Work out the finished part from the listing and answer in its coordinate system (mm). Round coordinates to 2 decimals unless told otherwise and drop trailing zeros. Order: outer loops, then holes, each group sorted by start corner. A loop starts at its lowest first (then second) coordinate and runs counter-clockwise, first axis right, second up. Notation, with made-up numbers: (14.25, 0.5) - (19.25, 0.5) arc R28 cw to (19.25, 20.5) - close; hole circle Ø10 at (50, 46.25). An arc over 180 degrees is marked (long way). Use CSV: the item, a comma, the result in double quotes.
from build123d import *

# Parameters (mm, degrees)
SKETCH1_R             = 20
SKETCH1_R_2           = 1
SKETCH1_R_3           = 5
BOSS_EXTRUDE1_DEPTH   = 9.35
M4X0_7_TAPPED_HOLE1_D = 3.3


with BuildPart() as part:
    # Sketch1 → Boss-Extrude1 (new body)
    with BuildSketch(Plane(origin=(0, 0, 0), x_dir=(1, 0, 0), z_dir=(0, 1, 0))):
        with Locations(Location((0, 0, 0), (0, 0, 270))):
            Circle(SKETCH1_R)
        with Locations(Location((0, 10, 0), (0, 0, 270))):
            Circle(SKETCH1_R_2, mode=Mode.SUBTRACT)
        with Locations(Location((8.660254038, 5, 0), (0, 0, 270))):
            Circle(SKETCH1_R_2, mode=Mode.SUBTRACT)
        with Locations(Location((8.660254038, -5, 0), (0, 0, 270))):
            Circle(SKETCH1_R_2, mode=Mode.SUBTRACT)
        with Locations(Location((0, -10, 0), (0, 0, 270))):
            Circle(SKETCH1_R_2, mode=Mode.SUBTRACT)
        with Locations(Location((-8.660254038, -5, 0), (0, 0, 270))):
            Circle(SKETCH1_R_2, mode=Mode.SUBTRACT)
        with Locations(Location((-8.660254038, 5, 0), (0, 0, 270))):
            Circle(SKETCH1_R_2, mode=Mode.SUBTRACT)
        with Locations(Location((0, 0, 0), (0, 0, 270))):
            Circle(SKETCH1_R_3, mode=Mode.SUBTRACT)
    extrude(amount=BOSS_EXTRUDE1_DEPTH)

    # M4x0.7 Tapped Hole1 (through all)
    with Locations(Plane(origin=(-8.660254038, 0, 5), x_dir=(0, 0, -1), z_dir=(0, -1, 0))):
        with Locations((0, 0), (-5, 8.660254038), (0, 17.320508076), (10, 17.320508076), (15, 8.660254038), (10, 0)):
            Hole(M4X0_7_TAPPED_HOLE1_D / 2)


solid = part.part
(1) Find the intervals of material crossed by L1, parallel to Z at x = 8.5, y = 1.75; L2, parallel to Z at x = 1.5, y = 5.5; L3, parallel to Z at x = 8, y = 5, in increasing order. Write a range as from..to.
Findings below:
L1,"z = -18.1..-6.64, -3.36..3.36, 6.64..18.1"
L2,"z = -19.94..-10.69, -9.31..-4.77, 4.77..9.31, 10.69..19.94"
L3,"z = -18.33..-6.51, -3.49..3.49, 6.51..18.33"
(2) Find section A-A (z = 0). Determine the outline of the cut face in (x, y).
Findings below:
outline,"(-20, 0) - (-5, 0) - (-5, 9.35) - (-20, 9.35) - close; (5, 0) - (20, 0) - (20, 9.35) - (5, 9.35) - close"
(3) Each of these flat-tipped pins is pushed along its axis until it touches: pin 1 (4 mm diameter, centred on x = -5, y = 6.5, fed in from +Z); pin 2 (1.5 mm diameter, centred on y = 5, z = 11, fed in from +X); pin 3 (1 mm diameter, centred on x = -2.5, y = 3, fed in from +Z). Where does it stop, or does it pass through?
Findings below:
pin 1,"stops at z = 19.77"
pin 2,"stops at x = 17.17"
pin 3,"stops at z = 19.9"
(4) Find section C-C (x = 8). Determine the outline of the cut face in (y, z), and give its area (3 significant figures).
Findings below:
outline,"(0, -18.33) - (9.35, -18.33) - (9.35, -6.51) - (0, -6.51) - close; (0, -3.49) - (9.35, -3.49) - (9.35, 3.49) - (0, 3.49) - close; (0, 6.51) - (9.35, 6.51) - (9.35, 18.33) - (0, 18.33) - close"
area,"286 mm²"
(5) The mould has two halves that part along Z. Classify faces 1 (the cylindrical face through (-19.524, 4.61, -4.336)), 2 (the cylindrical face through (-4.88, 4.61, -1.08)), 3 (the flat face through (-4, 9.35, 4)): released by +Z, released by -Z, zero draft, split by the parting line, or undercut.
Findings below:
face 1,"split by the parting line"
face 2,"undercut"
face 3,"zero draft"
(6) Find section D-D (y = 4). Determine the outline of the cut face in (x, z), and give its area (3 significant figures).
Findings below:
outline,"circle Ø40 at (0, 0); hole circle Ø3.3 at (-8.66, -5); hole circle Ø3.3 at (-8.66, 5); hole circle Ø10 at (0, 0); hole circle Ø3.3 at (0, -10); hole circle Ø3.3 at (0, 10); hole circle Ø3.3 at (8.66, -5); hole circle Ø3.3 at (8.66, 5)"
area,"1,130 mm²"
(7) Find section B-B (x = 0). Determine the outline of the cut face in (y, z).
Findings below:
outline,"(0, -20) - (9.35, -20) - (9.35, -11.65) - (0, -11.65) - close; (0, -8.35) - (9.35, -8.35) - (9.35, -5) - (0, -5) - close; (0, 5) - (9.35, 5) - (9.35, 8.35) - (0, 8.35) - close; (0, 11.65) - (9.35, 11.65) - (9.35, 20) - (0, 20) - close"
